Check sheet for the modelled part. Datum: model origin and axes. Units: mm. A direction names the side the tool comes from. Give positions to 0.01 mm unless a question says otherwise; leave off trailing zeros. Loops run counter-clockwise (first coordinate to the right, second up) from the corner with the lowest first, then second, coordinate; pieces in that order, holes last. Notation, with made-up numbers: M 39,29.25 L 45,29.25 A17 ccw 45,53.25 Z; hole C 75.5,-0.75 d4. An arc over 180 degrees is marked long. Use one line per item in the form item = value.
from build123d import *

# Parameters (mm, degrees)
EXTRUDE_1_DEPTH     = 140
SKETCH_2_R          = 1.65
CUT_EXTRUDE_1_DEPTH = 5
SKETCH_3_W          = 8
SKETCH_3_H          = 7.5
CUT_EXTRUDE_2_DEPTH = 146.701750161
SKETCH_4_W          = 10
SKETCH_4_H          = 8
CUT_EXTRUDE_3_DEPTH = 3.5
SKETCH_5_W          = 20
SKETCH_5_H          = 1.5
EXTRUDE_2_DEPTH     = 16
SKETCH_6_W          = 1.5
SKETCH_6_H          = 1.5
EXTRUDE_3_DEPTH     = 20
RIB_1_REACH         = 83.179
SKETCH_8_WALL_W     = 182.645829166
SKETCH_8_WALL_H     = 10
SKETCH_9_W          = 140
SKETCH_9_H          = 5
EXTRUDE_4_DEPTH     = 37
SKETCH_10_R         = 1.6
CUT_EXTRUDE_4_DEPTH = 5


with BuildPart() as part:
    # 草图1 → 凸台-拉伸1 (new body)
    with BuildSketch(Plane(origin=(0, 0, 0), x_dir=(0, 0, -1), z_dir=(1, 0, 0))):
        Polygon((-15, 27), (15, 27), (15, 22), (-8, 22), (-8, 17), (-8, -3), (-12, -3), (-12, -27), (-15, -27), align=None)
    extrude(amount=EXTRUDE_1_DEPTH)

    # 草图2 → 切除-拉伸1 (cut)
    with BuildSketch(Plane(origin=(0, 27, 0), x_dir=(1, 0, 0), z_dir=(0, 1, 0))):
        with Locations(Location((14, 3, 0), (0, 0, 270))):
            Circle(SKETCH_2_R)
        with Locations(Location((126, 3, 0), (0, 0, 270))):
            Circle(SKETCH_2_R)
    extrude(amount=-CUT_EXTRUDE_1_DEPTH, mode=Mode.SUBTRACT)

    # 草图3 → 切除-拉伸2 (cut, through all)
    with BuildSketch(Plane.XY.offset(15)):
        with Locations((10, 21.75)):
            Rectangle(SKETCH_3_W, SKETCH_3_H)
        with Locations((130, 21.75)):
            Rectangle(SKETCH_3_W, SKETCH_3_H)
    extrude(amount=-CUT_EXTRUDE_2_DEPTH, mode=Mode.SUBTRACT)

    # 草图4 → 切除-拉伸3 (cut)
    with BuildSketch(Plane.XZ.offset(-22)):
        with Locations((14, -3)):
            Rectangle(SKETCH_4_W, SKETCH_4_H)
        with Locations((126, -3)):
            Rectangle(SKETCH_4_W, SKETCH_4_H)
    extrude(amount=-CUT_EXTRUDE_3_DEPTH, mode=Mode.SUBTRACT)

    # 草图5 → 凸台-拉伸2 (add)
    with BuildSketch(Plane.XY.offset(15)):
        with Locations((70, -26.25)):
            Rectangle(SKETCH_5_W, SKETCH_5_H)
    extrude(amount=EXTRUDE_2_DEPTH)

    # 草图6 → 凸台-拉伸3 (add)
    with BuildSketch(Plane(origin=(80, 0, 0), x_dir=(0, 0, -1), z_dir=(1, 0, 0))):
        with Locations((-30.25, -24.75)):
            Rectangle(SKETCH_6_W, SKETCH_6_H)
    extrude(amount=-EXTRUDE_3_DEPTH)

    # 草图8 wall → 筋1 (add, up to next)
    with BuildSketch(Plane(origin=(70, -17.707455467, 19.784433865), x_dir=(0, -0.852193749384, 0.523226350168), z_dir=(0, 0.523226350168, 0.852193749384)), mode=Mode.PRIVATE) as rib_1_sk1:
        Rectangle(SKETCH_8_WALL_W, SKETCH_8_WALL_H)
    rib_1_tool1 = extrude(rib_1_sk1.sketch, amount=-RIB_1_REACH, mode=Mode.PRIVATE) - part.part
    add(rib_1_tool1.solids().sort_by_distance((70, -17.707455467, 19.784433865))[0])

    # 草图9 → 凸台-拉伸4 (add)
    with BuildSketch(Plane(origin=(0, 0, -15), x_dir=(-1, 0, 0), z_dir=(0, 0, -1))):
        with Locations((-70, 24.5)):
            Rectangle(SKETCH_9_W, SKETCH_9_H)
    extrude(amount=EXTRUDE_4_DEPTH)

    # 草图10 → 切除-拉伸4 (cut)
    with BuildSketch(Plane(origin=(0, 27, 0), x_dir=(1, 0, 0), z_dir=(0, 1, 0))):
        with Locations(Location((35.5, 46.5, 0), (0, 0, 270))):
            Circle(SKETCH_10_R)
        with Locations(Location((44.5, 46.5, 0), (0, 0, 270))):
            Circle(SKETCH_10_R)
        with Locations(Location((95.5, 46.5, 0), (0, 0, 270))):
            Circle(SKETCH_10_R)
        with Locations(Location((104.5, 46.5, 0), (0, 0, 270))):
            Circle(SKETCH_10_R)
    extrude(amount=-CUT_EXTRUDE_4_DEPTH, mode=Mode.SUBTRACT)


solid = part.part
1) Release check for a two-part mould opening along Y. For faces 6 (the face through (126, 23, 10)), 7 (the face through (14.496, 26.26, -1.426)), 8 (the face through (71, 27, -18)) record: pulls with the +Y half, pulls with the -Y half, needs draft (parallel to the pull), parting line crosses it, or undercut.
Evaluation:
face_6 = undercut
face_7 = needs draft
face_8 = pulls with the +Y half
2) Section check D-D (x = 104.5). Record the cut outline in (y, z), then the cut area to 3 significant figures.
Evaluation:
outline = M -27,12 L -3,12 L -3,8 L 22,8 L 22,-44.9 L 27,-44.9 L 27,15 L -27,15 Z; M 22,-52 L 27,-52 L 27,-48.1 L 22,-48.1 Z
area = 566 mm^2
3) Section check C-C (x = 41). Record the cut outline in (y, z).
Evaluation:
outline = M -27,12 L -3,12 L -3,8 L 22,8 L 22,-52 L 27,-52 L 27,15 L -27,15 Z
4) Set-up check for faces 1 (the face through (14, 24, -11)), 2 (the face through (80, -26, 23)), 3 (the face through (123, 24, -7)), 4 (the face through (69, -3, 10)), 5 (the face through (70, -25.5, 25)): record each of +Z, -Z, +X, -X, +Y, -Y from which the full face is reachable in a straight line by a thin tool's end or side.
Evaluation:
face_1 = +Z, -Y
face_2 = +Z, +X, +Y, -Y
face_3 = -Y
face_4 = -Z, +X, -X, -Y
face_5 = +Y
5) Scan lines: line 1 (Z direction, x = 126, y = 26); line 2 (Z direction, x = 104.5, y = 24.8); line 3 (Y direction, x = 133.5, z = -14). Record each from-to range of solid material in increasing order.
Evaluation:
line_1 = -52 to -4.65, -1.35 to 15
line_2 = -52 to -48.1, -44.9 to 15
line_3 = 25.5 to 27
6) Section check B-B (z = -3). Record the cut outline in (x, y), then the cut area to 3 significant figures.
Evaluation:
outline = M 0,22 L 6,22 L 6,25.5 L 12.35,25.5 L 12.35,27 L 0,27 Z; M 15.65,25.5 L 19,25.5 L 19,22 L 121,22 L 121,25.5 L 124.35,25.5 L 124.35,27 L 15.65,27 Z; M 127.65,25.5 L 134,25.5 L 134,22 L 140,22 L 140,27 L 127.65,27 Z
area = 599 mm^2
7) Section check A-A (x = 132). Record the cut outline in (y, z).
Evaluation:
outline = M -27,12 L -3,12 L -3,8 L 18,8 L 18,15 L -27,15 Z; M 22,-52 L 27,-52 L 27,15 L 25.5,15 L 25.5,-15 L 22,-15 Z
8) Depth check by flat-ended pin: pin 1 Ø4 at (y, z) = (22.5, -5.5) entering from -X; pin 2 Ø4 at (x, y) = (98, -14) entering from +Z; pin 3 Ø11.5 at (x, z) = (69, 25) entering from +Y; pin 4 Ø1.5 at (x, y) = (15.5, -3) entering from -Z. Enter the tip coordinate at first touch or a pass-through.
Evaluation:
pin_1 = 0
pin_2 = 15
pin_3 = -16.84
pin_4 = 8
